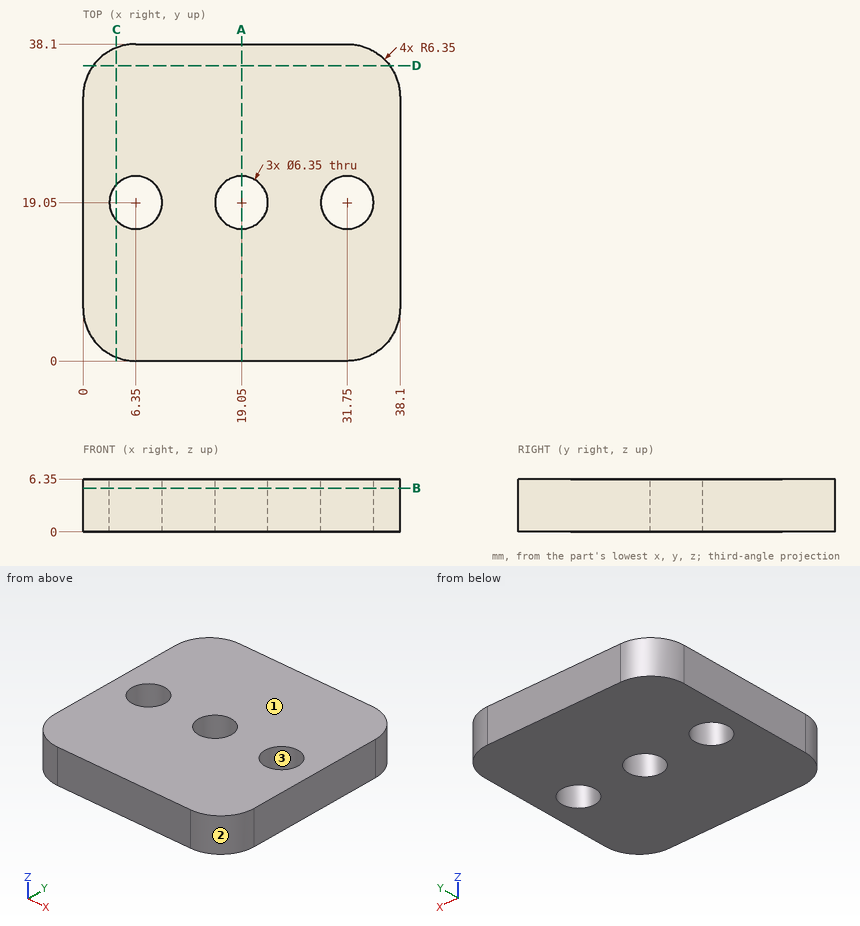
Study the drawing (mm; zero at the part's minimum x, y, z) and answer. Round coordinates to 2 decimals unless told otherwise and drop trailing zeros. Order: outer loops, then holes, each group sorted by start corner. A loop starts at its lowest first (then second) coordinate and runs counter-clockwise, first axis right, second up. Notation, with made-up numbers: (32.5, -29.5) -> (41.5, -29.5) arc R10 cw to (41.5, -11.5) -> close; hole circle Ø10 at (58, 81.25). An arc over 180 degrees is marked (long way). Answer as CSV lines item,"result". Start each with the question number.
(1) The part is cut by section A-A (x = 19.05). Determine the outline of the cut face in (y, z) (3 decimals), then the cut area to 3 significant figures.
(2) Find the intervals of material crossed by probe 1 along X at (y, z) = (19.05, 4.5) (3 decimals); probe 2 along Y at (x, z) = (19.05, 4.25) (3 decimals); probe 3 along X at (y, z) = (17, 0.75), in increasing order. Write a range as from..to.
(3) For a pull along Y with two mould halves and no side action, classify the marked faces 1, 2 and 3 as +Y half, -Y half, draft (parallel to the pull), parting line (faces both ways), or undercut.
(4) The part is cut by section B-B (z = 5.25). Determine the outline of the cut face in (x, y) (3 decimals).
(5) The part is cut by section C-C (x = 4). Determine the outline of the cut face in (y, z), then the cut area to 3 significant figures.
(6) The part is cut by section D-D (y = 35.5). Determine the outline of the cut face in (x, z).
(7) Flat-ended cylindrical pins translate along their axes: pin 1 Ø10 at (x, y) = (19.05, 19.05) entering from -Z; pin 2 Ø5 at (x, y) = (6.35, 19.05) entering from +Z. Find the tip coordinate at first contact, or state that the pin passes through.
Evaluation:
1,outline,"(0, 0) -> (15.875, 0) -> (15.875, 6.35) -> (0, 6.35) -> close; (22.225, 0) -> (38.1, 0) -> (38.1, 6.35) -> (22.225, 6.35) -> close"
1,area,"202 mm²"
2,probe 1,"0..3.175, 9.525..15.875, 22.225..28.575, 34.925..38.1"
2,probe 2,"0..15.875, 22.225..38.1"
2,probe 3,"0..3.93, 8.77..16.63, 21.47..29.33, 34.17..38.1"
3,face 1,"draft"
3,face 2,"-Y half"
3,face 3,"undercut"
4,outline,"(0, 6.35) arc R6.35 ccw to (6.35, 0) -> (31.75, 0) arc R6.35 ccw to (38.1, 6.35) -> (38.1, 31.75) arc R6.35 ccw to (31.75, 38.1) -> (6.35, 38.1) arc R6.35 ccw to (0, 31.75) -> close; hole circle Ø6.35 at (6.35, 19.05); hole circle Ø6.35 at (19.05, 19.05); hole circle Ø6.35 at (31.75, 19.05)"
5,outline,"(0.45, 0) -> (16.92, 0) -> (16.92, 6.35) -> (0.45, 6.35) -> close; (21.18, 0) -> (37.65, 0) -> (37.65, 6.35) -> (21.18, 6.35) -> close"
5,area,"209 mm²"
6,outline,"(1.23, 0) -> (36.87, 0) -> (36.87, 6.35) -> (1.23, 6.35) -> close"
7,pin 1,"z = 0"
7,pin 2,"through"
